Model file for the job. Use its own axes, mm. Round coordinates to 2 decimals unless told otherwise and drop trailing zeros. Write each loop counter-clockwise with the first axis right and the second up, starting at its lowest first coordinate (ties: lowest second). Pieces come first, ordered by that corner, then holes.
Autodesk Inventor part; units mm, degrees
ref_plane "YZ Plane" through (0, 0, 0) normal (1, 0, 0) x (0, 1, 0)
ref_plane "XZ Plane" through (0, 0, 0) normal (0, 1, 0) x (-1, 0, 0)
ref_plane "XY Plane" through (0, 0, 0) normal (0, 0, 1) x (1, 0, 0)
sketch "スケッチ1" plane through (0, 0, 0) normal (0, 0, 1) x (1, 0, 0)
  line L0 (24.05, 13.6) -> (24.05, 0.4)
  line L1 (24.05, 13.6) -> (37.25, 13.6)
  line L2 (37.25, 13.6) -> (37.25, 0.4)
  line L3 (56.5, 0.4) -> (37.25, 0.4)
  line L4 (56.5, 43.6) -> (56.5, 0.4)
  line L5 (2, 43.6) -> (56.5, 43.6)
  line L6 (2, 43.6) -> (2, 0.4)
  line L7 (24.05, 0.4) -> (2, 0.4)
  circle A0 centre (19.75, 30) radius 1.35
  circle A1 centre (51.75, 14) radius 1.35
  circle A2 centre (51.75, 30) radius 1.35
  circle A3 centre (19.75, 14) radius 1.35
  line L8 (2, 43.6) -> (56.5, 43.6)
  line L9 (56.5, 43.6) -> (56.5, 0.4)
  line L10 (56.5, 0.4) -> (2, 0.4)
  line L11 (2, 0.4) -> (2, 43.6)
  circle A4 centre (19.75, 14) radius 1.6
  circle A5 centre (19.75, 30) radius 1.6
  circle A6 centre (51.75, 30) radius 1.6
  circle A7 centre (51.75, 14) radius 1.6
  line L12 (-3.8486, -27.4677) -> (-13.8486, -27.4561)
  line L13 (34.25, -27.4677) -> (34.25, 112.5)
  line L14 (24.25, -27.4561) -> (24.25, 112.5)
  line L15 (24.25, 22) -> (34.25, 22)
  circle A8 centre (29.25, 22) radius 6.5
  circle A9 centre (29.25, 22) radius 40
  line L16 (2, 22) -> (-10.75, 22)
  line L17 (56.5, 22) -> (69.25, 22)
  line L18 (2, 22) -> (-4, 22)
  line L19 (-4, 22) -> (-4, 13)
  line L20 (-4, 13) -> (2, 13)
  line L21 (2, 13) -> (2, 22)
  line L22 (2, 22) -> (-4, 22)
  line L23 (-4, 22) -> (-4, 30)
  line L24 (-4, 30) -> (2, 30)
  line L25 (2, 30) -> (2, 22)
  line L26 (56.5, 22) -> (62.5, 22)
  line L27 (62.5, 22) -> (62.5, 14)
  line L28 (62.5, 14) -> (56.5, 14)
  line L29 (56.5, 14) -> (56.5, 22)
  line L30 (56.5, 22) -> (62.5, 22)
  line L31 (62.5, 22) -> (62.5, 30)
  line L32 (62.5, 30) -> (56.5, 30)
  line L33 (56.5, 30) -> (56.5, 22)
  circle A10 centre (-4, 13) radius 2
  circle A11 centre (-4, 30) radius 2
  circle A12 centre (62.5, 30) radius 2
  circle A13 centre (62.5, 14) radius 2
  line L34 (2, 43.6) -> (-4.4166, 43.6)
  line L35 (56.5, 43.6) -> (62.9166, 43.6)
  line L36 (2, 0.4) -> (-4.4166, 0.4)
  line L37 (56.5, 0.4) -> (62.9166, 0.4)
  point P0 (0, 0)
  point P1 (34.25, 112.5)
  point P2 (24.25, 112.5)
  point P3 (63.0326, 0.5819)
  point P4 (61.25, 46)
  point P5 (24.3716, 20.9038)
  point P6 (24.3687, 23.0832)
  point P7 (25.6996, 25.5206)
  point P8 (25.082, 19.2381)
  dimension "d7" = 80
  dimension "d0" = 3.2
  dimension "d1" = 3.2
  dimension "d2" = 3.2
  dimension "d3" = 3.2
  dimension "d6" = 13
  dimension "d8" = 6
  dimension "d9" = 9
  dimension "d10" = 6
  dimension "d11" = 4
  dimension "d12" = 4
  dimension "d13" = 4
  dimension "d14" = 4
extrude "押し出し1" add sketch "スケッチ1" along normal blind 1.5 contours L1 L14 L10 L0 | L0 L7 L6 L5 L14 A8 L1 | L14 A8 L13 L1 | L1 L13 L10 L14 | L36 A9 L16 L19 A10 L20 L6 | L13 A8 L5 L4 L3 L2 L1 | L1 L2 L10 L13 | L20 A10 L19 L16 L6 | L14 L5 L13 A8 | L16 L23 A11 L24 L6 | A9 L34 L6 L24 A11 L23 L16 | L4 L28 A13 L27 L17 A9 L37 | L4 L17 L27 A13 L28 | L17 L31 A12 L32 L4 L35 A9 | L4 L32 A12 L31 L17
sketch "スケッチ2" plane through (0, 0, 1.5) normal (0, 0, 1) x (1, 0, 0)
  point P0 (0, 0)
1) Cut at C-C on x = 19.75. List the corners of the cut face in (y, z), and give its area (3 significant figures).
2) Wall check: probe 1 along Y at (x, z) = (62.5, 1.1); probe 2 along Y at (x, z) = (19.75, 0.7); probe 3 along X at (y, z) = (13, 0.95). Give the ranges that are in metal, low to high.
3) Cut at A-A on x = 29.25. List the corners of the cut face in (y, z).
4) Cut at B-B on y = 22. List the corners of the cut face in (x, z), and give its area (4 significant figures).
5) Pull direction X, two halves, no side cores. Call faces 1 (the face through (-10.75, 21.68, 0.74)), 2 (the face through (69.25, 22.32, 0.74)), 3 (the face through (30, 0.4, 1)), 4 (the face through (62.066, 31.952, 0.74)): released by +X, released by -X, zero draft, split by the parting line, or undercut.
6) Cut at D-D on z = 1. Give the number of separate pieces and of enclosed holes in the cut face, and give its area (3 significant figures).
Result sheet:
1. outline: (0.4, 0) - (12.4, 0) - (12.4, 1.5) - (0.4, 1.5) - close; (15.6, 0) - (28.4, 0) - (28.4, 1.5) - (15.6, 1.5) - close; (31.6, 0) - (43.6, 0) - (43.6, 1.5) - (31.6, 1.5) - close
1. area: 55.2 mm2
2. probe 1: y = 0.4 to 12, 16 to 28, 32 to 43.6
2. probe 2: y = 0.4 to 12.4, 15.6 to 28.4, 31.6 to 43.6
2. probe 3: x = -9.72 to -6, -2 to 18.5, 21 to 50.5, 53 to 60.77, 64.23 to 68.22
3. outline: (0.4, 0) - (15.5, 0) - (15.5, 1.5) - (0.4, 1.5) - close; (28.5, 0) - (43.6, 0) - (43.6, 1.5) - (28.5, 1.5) - close
4. outline: (-10.75, 0) - (22.75, 0) - (22.75, 1.5) - (-10.75, 1.5) - close; (35.75, 0) - (69.25, 0) - (69.25, 1.5) - (35.75, 1.5) - close
4. area: 100.5 mm2
5. face 1: released by -X
5. face 2: released by +X
5. face 3: zero draft
5. face 4: undercut
6. separate pieces: 1
6. enclosed holes: 9
6. area: 3,060 mm2
